```python
from build123d import *


with BuildPart() as part:
    # Sketch1 → Revolve1 (revolve)
    with BuildSketch(Plane.XY, mode=Mode.PRIVATE) as revolve1_sk:
        Polygon((0, 0), (0, 0.6223), (1.9304, 0.6223), (2.6797, 1.3716), (4.084417728, 1.3716), (4.2164, 1.4478), (4.2164, 1.3716), (5.2324, 1.3716), (5.2324, 1.7526), (7.1374, 1.7526), (7.1374, 0), align=None)
    revolve(revolve1_sk.sketch.rotate(Axis((-2.173675745, 0, 0), (1, 0, 0)), 90), axis=Axis((-2.173675745, 0, 0), (1, 0, 0)))

    # Sketch2 → Cut-Revolve1 (revolve, cut)
    with BuildSketch(Plane.XY, mode=Mode.PRIVATE) as cut_revolve1_sk:
        with BuildLine():
            Line((0.6223, 0.6223), (-0.23767542, 0.6223))
            Line((-0.23767542, 0.6223), (-0.23767542, 0))
            Line((-0.23767542, 0), (0, 0))
            ThreePointArc((0, 0), (0.18226745, 0.44003255), (0.6223, 0.6223))
        make_face()
    revolve(cut_revolve1_sk.sketch.rotate(Axis((-2.173675745, 0, 0), (1, 0, 0)), 90), axis=Axis((-2.173675745, 0, 0), (1, 0, 0)), mode=Mode.SUBTRACT)


solid = part.part
```
For this review, take the finished solid that the model builds, in its own axes (mm). Give positions to 0.01 mm unless a question says otherwise; leave off trailing zeros. Loops run counter-clockwise (first coordinate to the right, second up) from the corner with the lowest first, then second, coordinate; pieces in that order, holes last. Notation, with made-up numbers: M -38.75,-2.75 L 3.25,-2.75 A23 ccw 3.25,17.25 Z; hole C 67.25,15 d8. An arc over 180 degrees is marked long. One line per item, written item: value. Start each with the question number.
Q1. For L1, parallel to X at y = -1.5, z = -0.3; L2, parallel to Z at x = 4, y = -0.3; L3, parallel to Y at x = 3, z = -0.4, list the stretches that pass through material, from the lowest coordinate up.
Q2. Draft analysis for pull direction X (two halves, no side actions). For faces 1 (the face through (7.137, 0, 0)), 2 (the face through (6.2, -0.53, 1.67)), 3 (the face through (4.73, -0.06, -1.37)), state which applies: released by +X, released by -X, zero draft, split by the parting line, or undercut.
Q3. Add section D-D (x = 1.25). Give the boundary of the cut face in (y, z).
Q4. Add section C-C (x = 3). Give the boundary of the cut face in (y, z).
Q5. Add section A-A (y = 0). Give the boundary of the cut face in (x, z), and give its area (3 significant figures).
Reply:
1. L1: 5.23 to 7.14
1. L2: -1.34 to 1.34
1. L3: -1.31 to 1.31
2. face 1: released by +X
2. face 2: zero draft
2. face 3: undercut
3. outline: C 0,0 d1.24
4. outline: C 0,0 d2.74
5. outline: M 0.62,-0.62 L 1.93,-0.62 L 2.68,-1.37 L 4.08,-1.37 L 4.22,-1.45 L 4.22,-1.37 L 5.23,-1.37 L 5.23,-1.75 L 7.14,-1.75 L 7.14,1.75 L 5.23,1.75 L 5.23,1.37 L 4.22,1.37 L 4.22,1.45 L 4.08,1.37 L 2.68,1.37 L 1.93,0.62 L 0.62,0.62 A0.62 ccw Z
5. area: 17.4 mm²
